```python
from build123d import *

# Parameters (mm, degrees)
PAD_DEPTH       = 14
SKETCH001_R     = 2.5
POCKET_DEPTH    = 33.501
FILLET_R        = 2
FILLET001_R     = 1
CHAMFER_SIZE    = 1
CHAMFER001_SIZE = 1
SKETCH002_R     = 1.5
POCKET001_DEPTH = 30.001
SKETCH003_R     = 3.5
POCKET002_DEPTH = 4
FILLET002_R     = 0.5


with BuildPart() as part:
    # Sketch → Pad (new body)
    with BuildSketch(Plane.XY):
        with BuildLine():
            Line((-20, -21), (-13.5, -21))
            Line((-13.5, -9), (-13.5, -21))
            Line((-13.5, -9), (13.5, -9))
            Line((13.5, -9), (13.5, -0.5))
            Line((3.968627, -0.5), (13.5, -0.5))
            ThreePointArc((3.968627, 0.5), (-4, 0), (3.968627, -0.5))
            Line((3.968627, 0.5), (13.5, 0.5))
            Line((13.5, 0.5), (13.5, 9))
            Line((13.5, 9), (-13.5, 9))
            Line((-13.5, 9), (-13.5, 21))
            Line((-13.5, 21), (-20, 21))
            Line((-20, 21), (-20, -21))
        make_face()
    extrude(amount=PAD_DEPTH)

    # Sketch001 (on Face6 of Pad) → Pocket (cut, through all)
    with BuildSketch(Plane(origin=(-20, 0, 0), x_dir=(0, -1, 0), z_dir=(-1, 0, 0))):
        with Locations((-16, 7)):
            Circle(SKETCH001_R)
        with Locations((16, 7)):
            Circle(SKETCH001_R)
    extrude(amount=-POCKET_DEPTH, mode=Mode.SUBTRACT)

    # Fillet
    fillet_edges = [part.edges().sort_by_distance(p)[0] for p in [
        (-20, 21, 7),
        (-20, -21, 7),
    ]]
    fillet(fillet_edges, radius=FILLET_R)

    # Fillet001
    fillet001_edges = [part.edges().sort_by_distance(p)[0] for p in [
        (13.5, 9, 7),
        (13.5, -9, 7),
    ]]
    fillet(fillet001_edges, radius=FILLET001_R)

    # Chamfer
    chamfer_edges = [part.edges().sort_by_distance(p)[0] for p in [
        (-4, 0, 14),
    ]]
    chamfer(chamfer_edges, length=CHAMFER_SIZE)

    # Chamfer001
    chamfer001_edges = [part.edges().sort_by_distance(p)[0] for p in [
        (-4, 0, 0),
    ]]
    chamfer(chamfer001_edges, length=CHAMFER001_SIZE)

    # Sketch002 (on Face11 of Chamfer001) → Pocket001 (cut, through all)
    with BuildSketch(Plane(origin=(0, 9, 0), x_dir=(-1, 0, 0), z_dir=(0, 1, 0))):
        with Locations((-9, 7)):
            Circle(SKETCH002_R)
    extrude(amount=-POCKET001_DEPTH, mode=Mode.SUBTRACT)

    # Sketch003 (on Face15 of Pocket001) → Pocket002 (cut)
    with BuildSketch(Plane.XZ.offset(9)):
        with Locations((9, 7)):
            Circle(SKETCH003_R)
    extrude(amount=-POCKET002_DEPTH, mode=Mode.SUBTRACT)

    # Fillet002
    fillet002_edges = [part.edges().sort_by_distance(p)[0] for p in [
        (-0.5, -9, 14),
        (-0.5, -9, 0),
        (-0.5, 9, 14),
        (-0.5, 9, 0),
        (-13.5, -15, 0),
        (-13.5, -15, 14),
        (-13.5, 15, 0),
        (-13.5, -21, 7),
        (-13.5, 21, 7),
        (-13.5, 15, 14),
        (-15.75, 21, 14),
        (-15.75, 21, 0),
        (-15.75, -21, 0),
        (-15.75, -21, 14),
        (13.5, -4.25, 0),
        (13.5, 4.25, 0),
        (13.5, -4.25, 14),
        (13.5, 4.25, 14),
        (13.207107, -8.707107, 14),
        (13.207107, 8.707107, 14),
        (13.207107, 8.707107, 0),
        (13.207107, -8.707107, 0),
    ]]
    fillet(fillet002_edges, radius=FILLET002_R)


solid = part.part
```
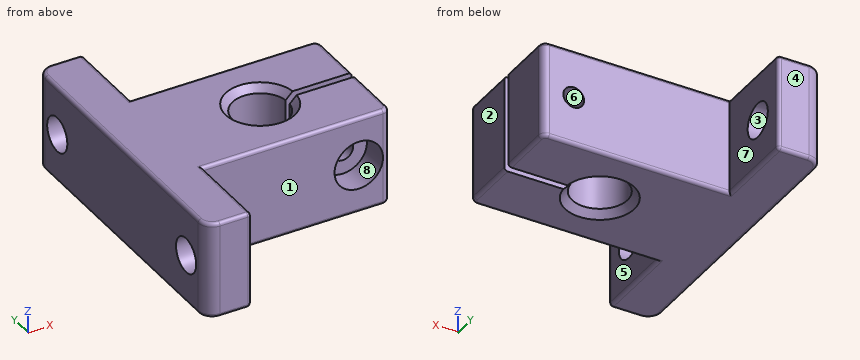
CAD build for the part. Positions are in the model's coordinates, mm. Face numbers are marked on the shaded views. A direction names the side the tool comes from. Round coordinates to 2 decimals unless told otherwise and drop trailing zeros. Order: outer loops, then holes, each group sorted by start corner. A loop starts at its lowest first (then second) coordinate and runs counter-clockwise, first axis right, second up. Notation, with made-up numbers: (68.5, 20.25) - (127.5, 20.25) arc R26 ccw to (127.5, 46.25) - close; hole circle Ø7 at (-16.75, 84). An arc over 180 degrees is marked (long way). Use CSV: the item, a comma, the result in double quotes. Start each with the question number.
1) Saw through at B-B (y = -7). List the corners of the cut face in (x, z).
2) Two-plate mould, pull along Y, no slides. Class the marked faces 1, 2, 3 and 4: pulls with the +Y half, pulls with the -Y half, needs draft (parallel to the pull), parting line crosses it, or undercut.
3) Tool access for the marked faces 5, 6, 7 and 8: list every direction of +Z, -Z, +X, -X, +Y, -Y with a clear straight run to the whole face (end or side of a thin tool).
4) Pin check, flat tips, straight feed: pin 1 Ø1 at (x, z) = (-4, 7.5) entering from -Y; pin 2 Ø4 at (x, z) = (9, 7) entering from -Y; pin 3 Ø6 at (y, z) = (16, 7) entering from -X; pin 4 Ø1 at (x, z) = (-2.5, 4) entering from +Y. Stop position of each tip, or through.
5) Saw through at D-D (y = -16). List the corners of the cut face in (x, z), and give its area (3 significant figures).
6) Wall check: L1, parallel to Y at x = 4.5, z = 5.75; L2, parallel to X at y = 3, z = 6; L3, parallel to Z at x = -17, y = 16. Give the ranges that are in metal, low to high. Write a range as [from, to].
7) Saw through at C-C (z = 5). Count the separate pieces of the cut face and the enclosed holes in it, and give its area (3 significant figures).
8) Saw through at A-A (x = 0). List the corners of the cut face in (y, z), and give its area (3 significant figures).
Values follow:
1,outline,"(-20, 0.5) arc R0.5 ccw to (-19.5, 0) - (13, 0) arc R0.5 ccw to (13.5, 0.5) - (13.5, 13.5) arc R0.5 ccw to (13, 14) - (-19.5, 14) arc R0.5 ccw to (-20, 13.5) - close; hole circle Ø7 at (9, 7)"
2,face 1,"pulls with the -Y half"
2,face 2,"needs draft"
2,face 3,"undercut"
2,face 4,"pulls with the +Y half"
3,face 5,"+Z, -Z, +X, -Y"
3,face 6,"+Y, -Y"
3,face 7,"+Z, -Z, +X, +Y"
3,face 8,"-Y"
4,pin 1,"stops at y = -9"
4,pin 2,"stops at y = -5"
4,pin 3,"stops at x = -20"
4,pin 4,"stops at y = 9"
5,outline,"(-20, 0.5) arc R0.5 ccw to (-19.5, 0) - (-14, 0) arc R0.5 ccw to (-13.5, 0.5) - (-13.5, 4.5) - (-20, 4.5) - close; (-20, 9.5) - (-13.5, 9.5) - (-13.5, 13.5) arc R0.5 ccw to (-14, 14) - (-19.5, 14) arc R0.5 ccw to (-20, 13.5) - close"
5,area,"58.3 mm2"
6,L1,"y = [-9, -0.5], [0.5, 9]"
6,L2,"x = [-20, -2.65], [2.65, 7.88], [10.12, 13.5]"
6,L3,"z = [0, 4.5], [9.5, 14]"
7,separate pieces,"3"
7,enclosed holes,"0"
7,area,"635 mm2"
8,outline,"(-9, 0.5) arc R0.5 ccw to (-8.5, 0) - (-5, 0) - (-4, 1) - (-4, 13) - (-5, 14) - (-8.5, 14) arc R0.5 ccw to (-9, 13.5) - close; (4, 1) - (5, 0) - (8.5, 0) arc R0.5 ccw to (9, 0.5) - (9, 13.5) arc R0.5 ccw to (8.5, 14) - (5, 14) - (4, 13) - close"
8,area,"138 mm2"
